from build123d import *

# Parameters (mm, degrees)
SKETCH1_R           = 101.6
BOSS_EXTRUDE1_DEPTH = 50.8
BOSS_EXTRUDE2_DEPTH = 101.6
CHAMFER1_SIZE       = 7.62
SKETCH3_R           = 38.1
CUT_EXTRUDE1_DEPTH  = 102.6


with BuildPart() as part:
    # Sketch1 → Boss-Extrude1 (new body, symmetric)
    with BuildSketch(Plane.XY):
        Circle(SKETCH1_R)
    extrude(amount=BOSS_EXTRUDE1_DEPTH, both=True)

    # Sketch2 → Boss-Extrude2 (add, through all)
    with BuildSketch(Plane.XY.offset(50.8)):
        with BuildLine():
            Line((74.498522628, 103.635226281), (52.501477372, 116.335226281))
            Line((52.501477372, 116.335226281), (39.403039848, 93.648066989))
            ThreePointArc((39.403039848, 93.648066989), (50.8, 87.988181024), (61.400085104, 80.948066989))
            Line((61.400085104, 80.948066989), (74.498522628, 103.635226281))
        make_face()
        with BuildLine():
            Line((12.7, 100.803124952), (12.7, 127))
            Line((12.7, 127), (-12.7, 127))
            Line((-12.7, 127), (-12.7, 100.803124952))
            ThreePointArc((-12.7, 100.803124952), (0, 101.6), (12.7, 100.803124952))
        make_face()
        with BuildLine():
            Line((116.335226281, 52.501477372), (103.635226281, 74.498522628))
            Line((103.635226281, 74.498522628), (80.948066989, 61.400085104))
            ThreePointArc((80.948066989, 61.400085104), (87.988181024, 50.8), (93.648066989, 39.403039848))
            Line((93.648066989, 39.403039848), (116.335226281, 52.501477372))
        make_face()
        with BuildLine():
            Line((127, -12.7), (127, 12.7))
            Line((127, 12.7), (100.803124952, 12.7))
            ThreePointArc((100.803124952, 12.7), (101.6, 0), (100.803124952, -12.7))
            Line((100.803124952, -12.7), (127, -12.7))
        make_face()
        with BuildLine():
            Line((103.635226281, -74.498522628), (116.335226281, -52.501477372))
            Line((116.335226281, -52.501477372), (93.648066989, -39.403039848))
            ThreePointArc((93.648066989, -39.403039848), (87.988181024, -50.8), (80.948066989, -61.400085104))
            Line((80.948066989, -61.400085104), (103.635226281, -74.498522628))
        make_face()
        with BuildLine():
            Line((52.501477372, -116.335226281), (74.498522628, -103.635226281))
            Line((74.498522628, -103.635226281), (61.400085104, -80.948066989))
            ThreePointArc((61.400085104, -80.948066989), (50.8, -87.988181024), (39.403039848, -93.648066989))
            Line((39.403039848, -93.648066989), (52.501477372, -116.335226281))
        make_face()
        with BuildLine():
            Line((-12.7, -127), (12.7, -127))
            Line((12.7, -127), (12.7, -100.803124952))
            ThreePointArc((12.7, -100.803124952), (0, -101.6), (-12.7, -100.803124952))
            Line((-12.7, -100.803124952), (-12.7, -127))
        make_face()
        with BuildLine():
            Line((-74.498522628, -103.635226281), (-52.501477372, -116.335226281))
            Line((-52.501477372, -116.335226281), (-39.403039848, -93.648066989))
            ThreePointArc((-39.403039848, -93.648066989), (-50.8, -87.988181024), (-61.400085104, -80.948066989))
            Line((-61.400085104, -80.948066989), (-74.498522628, -103.635226281))
        make_face()
        with BuildLine():
            Line((-116.335226281, -52.501477372), (-103.635226281, -74.498522628))
            Line((-103.635226281, -74.498522628), (-80.948066989, -61.400085104))
            ThreePointArc((-80.948066989, -61.400085104), (-87.988181024, -50.8), (-93.648066989, -39.403039848))
            Line((-93.648066989, -39.403039848), (-116.335226281, -52.501477372))
        make_face()
        with BuildLine():
            Line((-127, 12.7), (-127, -12.7))
            Line((-127, -12.7), (-100.803124952, -12.7))
            ThreePointArc((-100.803124952, -12.7), (-101.6, 0), (-100.803124952, 12.7))
            Line((-100.803124952, 12.7), (-127, 12.7))
        make_face()
        with BuildLine():
            Line((-103.635226281, 74.498522628), (-116.335226281, 52.501477372))
            Line((-116.335226281, 52.501477372), (-93.648066989, 39.403039848))
            ThreePointArc((-93.648066989, 39.403039848), (-87.988181024, 50.8), (-80.948066989, 61.400085104))
            Line((-80.948066989, 61.400085104), (-103.635226281, 74.498522628))
        make_face()
        with BuildLine():
            Line((-52.501477372, 116.335226281), (-74.498522628, 103.635226281))
            Line((-74.498522628, 103.635226281), (-61.400085104, 80.948066989))
            ThreePointArc((-61.400085104, 80.948066989), (-50.8, 87.988181024), (-39.403039848, 93.648066989))
            Line((-39.403039848, 93.648066989), (-52.501477372, 116.335226281))
        make_face()
    extrude(amount=-BOSS_EXTRUDE2_DEPTH)

    # Chamfer1
    chamfer1_edges = [part.edges().sort_by_distance(p)[0] for p in [
        (-127, -12.7, 0),
        (-127, 12.7, 0),
        (-116.335226281, 52.501477372, 0),
        (-103.635226281, 74.498522628, 0),
        (-74.498522628, 103.635226281, 0),
        (-52.501477372, 116.335226281, 0),
        (52.501477372, 116.335226281, 0),
        (74.498522628, 103.635226281, 0),
        (103.635226281, 74.498522628, 0),
        (116.335226281, 52.501477372, 0),
        (127, 12.7, 0),
        (127, -12.7, 0),
        (116.335226281, -52.501477372, 0),
        (103.635226281, -74.498522628, 0),
        (74.498522628, -103.635226281, 0),
        (52.501477372, -116.335226281, 0),
        (12.7, -127, 0),
        (-12.7, -127, 0),
        (-12.7, 127, 0),
        (12.7, 127, 0),
        (-52.501477372, -116.335226281, 0),
        (-74.498522628, -103.635226281, 0),
        (-103.635226281, -74.498522628, 0),
        (-116.335226281, -52.501477372, 0),
    ]]
    chamfer(chamfer1_edges, length=CHAMFER1_SIZE)

    # Sketch3 → Cut-Extrude1 (cut, through all)
    with BuildSketch(Plane.XY.offset(50.8)):
        Circle(SKETCH3_R)
    extrude(amount=-CUT_EXTRUDE1_DEPTH, mode=Mode.SUBTRACT)


solid = part.part
Verification items for the finished model (mm, model axes). A direction names the side the tool comes from. Round coordinates to 2 decimals unless told otherwise and drop trailing zeros. Order: outer loops, then holes, each group sorted by start corner. A loop starts at its lowest first (then second) coordinate and runs counter-clockwise, first axis right, second up.
1. Release check for a two-part mould opening along X. For faces 1 (the flat face through (-111.15, -53.97, 0.71)), 2 (the flat face through (-53.97, 111.15, 0.71)), 3 (the flat face through (123.14, 8.94, 0.71)) record: +X half, -X half, draft (parallel to the pull), parting line (faces both ways), or undercut.
Final values:
face 1: -X half
face 2: undercut
face 3: +X half
2. Go/stop test with flat-tipped pins: P1, Ø20.5, axis at y = 113.5, z = 2.5, coming from the -X side; P2, Ø5.5, axis at x = 112, z = 23, coming from the -Y side; P3, Ø10, axis at y = -36.5, z = 25, coming from the +X side. Record where each tip stops, or that it passes through.
Final values:
P1: stops at x = -69.02
P2: stops at y = -64.77
P3: stops at x = 97.28
3. Section check C-C on x = -75.5. Record the cut outline in (y, z).
Final values:
outline: (-67.99, -50.8) - (67.99, -50.8) - (67.99, 50.8) - (-67.99, 50.8) - close
4. Thickness scan on L1, parallel to Y at x = 0, z = 8; L2, parallel to Y at x = -104.5, z = 18.5; L3, parallel to X at y = 107.5, z = -38.5. Record the ranges inside material, lowest first.
Final values:
L1: y = -127 to -38.1, 38.1 to 127
L2: y = -68.69 to -45.67, -12.7 to 12.7, 45.67 to 68.69
L3: x = -67.8 to -47.4, -12.7 to 12.7, 47.4 to 67.8
5. Access from +Z, -Z, +X, -X, +Y, -Y to the whole of each face (thin tool, end or side, straight path). Record for faces 4 (the cylindrical face through (-71.705, 71.979, 0.711)), 5 (the flat face through (109.95, -63.56, 0.71)), 6 (the flat face through (65.98, 88.88, 0.71)), 7 (the flat face through (-101.579, -43.982, 0.711)).
Final values:
face 4: +Z, -Z
face 5: +Z, -Z, +X, -Y
face 6: +Z, -Z, +X
face 7: +Z, -Z, -X
6. Section check A-A on x = 0. Record the cut outline in (y, z).
Final values:
outline: (-127, -50.8) - (-38.1, -50.8) - (-38.1, 50.8) - (-127, 50.8) - close; (38.1, -50.8) - (127, -50.8) - (127, 50.8) - (38.1, 50.8) - close
